Read the model definition and answer for the solid it produces. Units are mm, in the model's axes. Give positions to 0.01 mm unless a question says otherwise; leave off trailing zeros. Order: outer loops, then holes, each group sorted by start corner. A loop starts at its lowest first (then second) coordinate and runs counter-clockwise, first axis right, second up.
Item 1: The mould has two halves that part along Z. Classify faces 1 (the face through (-0.69, -7.65, -3.1)), 2 (the face through (0, -6.35, 0)): +Z half, -Z half, draft (parallel to the pull), parting line (faces both ways), or undercut.
Item 2: A cutting plane is placed at A-A (z = 0). Write down the section's boundary in (x, y) (3 decimals).
Item 3: A cutting plane is placed at B-B (x = 0). Write down the section's boundary in (y, z) (3 decimals).
Item 4: Find the intervals of material crossed by line 1 along Z through (x, y) = (0, -7.2) (3 decimals); line 2 along X through (y, z) = (-7.7, 0) (3 decimals); line 3 along X through (y, z) = (-7.3, 0) (3 decimals), in increasing order.
Item 5: A cutting plane is placed at D-D (z = 7). Write down the section's boundary in (x, y).
Item 6: Given pin 1 Ø1.9 at (x, z) = (-0.5, -1.5) entering from -Y; pin 2 Ø5 at (y, z) = (-3.5, 4.5) entering from +X; pin 3 Ø4 at (x, z) = (-6, -3) entering from +Y, each flat-ended and moving along its own axis, determine where each tip first touches the part or whether it passes through.
Item 7: A cutting plane is placed at C-C (y = 1). Write down the section's boundary in (x, z).
from build123d import *

# Parameters (mm, degrees)
F3_R     = 3.175
F4_DEPTH = 25.4


with BuildPart() as f1:
    # F0 (on Top) → F1 (revolve)
    with BuildSketch(Plane.XY):
        with BuildLine():
            Line((0, -9.525), (0, 9.525))
            ThreePointArc((0, 9.525), (-9.525, 0), (0, -9.525))
        make_face()
    revolve(axis=Axis((0, 0, 0), (0, -1, 0)))


with BuildPart() as f4:
    # F3 (on offset) → F4 (new body)
    with BuildSketch(Plane.XZ.offset(6.35)):
        Circle(F3_R)
    extrude(amount=F4_DEPTH)


with BuildPart() as f1_1:
    add(f1.part)

    # F5: cut F4
    add(f4.part, mode=Mode.SUBTRACT)


solid = f1_1.part
Response values:
1. face 1: undercut
1. face 2: undercut
2. outline: (-3.175, -8.98) - (-3.175, -6.35) - (3.175, -6.35) - (3.175, -8.98) arc R9.525 ccw (long way) to start
3. outline: (-8.98, -3.175) arc R9.525 ccw (long way) to (-8.98, 3.175) - (-6.35, 3.175) - (-6.35, -3.175) - close
4. line 1: z = -6.236 to -3.175, 3.175 to 6.236
4. line 2: x = -5.607 to -3.175, 3.175 to 5.607
4. line 3: x = -6.118 to -3.175, 3.175 to 6.118
5. outline: circle Ø12.92 at (0, 0)
6. pin 1: stops at y = -6.35
6. pin 2: stops at x = 8.97
6. pin 3: stops at y = 8.28
7. outline: circle Ø18.94 at (0, 0)
